Build history of the part. All positions in model axes, mm. A direction names the side the tool comes from. Give positions to 0.01 mm unless a question says otherwise; leave off trailing zeros. Answer as CSV lines item,"result".
from build123d import *

# Parameters (mm, degrees)
SKETCH1_W             = 82
SKETCH1_H             = 50
BOSS_EXTRUDE1_DEPTH   = 16
CHAMFER1_SIZE         = 1.5
M4_TAPPED_HOLE1_D     = 3.3
M4_TAPPED_HOLE1_DEPTH = 6
M4_TAPPED_HOLE1_TIP   = 0.991420021


with BuildPart() as part:
    # Sketch1 → Boss-Extrude1 (new body)
    with BuildSketch(Plane(origin=(0, 0, 0), x_dir=(1, 0, 0), z_dir=(0, 1, 0))):
        Rectangle(SKETCH1_W, SKETCH1_H)
    extrude(amount=BOSS_EXTRUDE1_DEPTH)

    # Chamfer1
    chamfer1_edges = [part.edges().sort_by_distance(p)[0] for p in [
        (41, 16, 0),
        (0, 16, -25),
        (-41, 16, 0),
        (0, 16, 25),
    ]]
    chamfer(chamfer1_edges, length=CHAMFER1_SIZE)

    # M4 Tapped Hole1
    with Locations(Plane(origin=(0, 16, 0), x_dir=(1, 0, 0), z_dir=(0, 1, 0))):
        with Locations((-19, 12.5), (19, 12.5), (19, -12.5), (-19, -12.5)):
            Hole(M4_TAPPED_HOLE1_D / 2, depth=M4_TAPPED_HOLE1_DEPTH)
            with Locations((0, 0, -(M4_TAPPED_HOLE1_DEPTH + M4_TAPPED_HOLE1_TIP / 2))):  # 118° drill point
                Cone(0, M4_TAPPED_HOLE1_D / 2, M4_TAPPED_HOLE1_TIP, mode=Mode.SUBTRACT)


solid = part.part
Item 1: Probe line 1 along Z through (x, y) = (-19, 14.2); line 2 along X through (y, z) = (12.3, 12.5); line 3 along X through (y, z) = (15.25, -5.5). List the from-to ranges inside material, lowest first. Write a range as from..to.
Geometry says:
line 1,"z = -25..-14.15, -10.85..10.85, 14.15..25"
line 2,"x = -41..-20.65, -17.35..17.35, 20.65..41"
line 3,"x = -40.25..40.25"
Item 2: Drop flat-ended pins along their axis: pin 1 (3 mm diameter, centred on x = -30.5, z = -2, fed in from -Y); pin 2 (2 mm diameter, centred on x = -19, z = 12.5, fed in from +Y); pin 3 (2.5 mm diameter, centred on x = -19, z = -12.5, fed in from +Y). Give the stop position or say it passes through.
Geometry says:
pin 1,"stops at y = 0"
pin 2,"stops at y = 9.61"
pin 3,"stops at y = 9.76"
Item 3: 3-axis set-ups, long thin cutter, end or side, ignore diameter. For faces 5 (the flat face through (-40.2, 15.3, 0.3)), 6 (the cylindrical face through (-17.69, 12.96, 13.5)): which of +Z, -Z, +X, -X, +Y, -Y reach the whole face in a straight line?
Geometry says:
face 5,"+Z, -Z, -X, +Y"
face 6,"+Y"
Item 4: Pull direction X, two halves, no side cores. Call faces 1 (the flat face through (40.2, 15.3, 0.3)), 2 (the cylindrical face through (-17.69, 12.96, -11.5)), 3 (the flat face through (-41, 7, 0)), 4 (the flat face through (-1, 16, 0)): released by +X, released by -X, zero draft, split by the parting line, or undercut.
Geometry says:
face 1,"released by +X"
face 2,"undercut"
face 3,"released by -X"
face 4,"zero draft"
